Can you work these out from the model? Positions are in its coordinate system, mm. A direction names the side the tool comes from. Give positions to 0.01 mm unless a question says otherwise; leave off trailing zeros. Order: outer loops, then holes, each group sorted by start corner. A loop starts at its lowest first (then second) coordinate and runs counter-clockwise, first axis right, second up.
```python
from build123d import *

# Parameters (mm, degrees)
F2_R = 3.875


with BuildPart() as f3:
    # F3: sweep along a path in F0
    with BuildLine(Plane.XZ) as f3_path:
        Line((18, 62), (18, 16.4454190283))
        ThreePointArc((18, 16.4454190283), (17.4915763011, 14.2486617975), (16.0697030676, 12.4986579414))
        Line((16.0697030676, 12.4986579414), (3.0697030676, 2.3875468303))
        ThreePointArc((3.0697030676, 2.3875468303), (0, 1.3343079172), (-3.0697030676, 2.3875468303))
        Line((-3.0697030676, 2.3875468303), (-16.0697030676, 12.4986579414))
        ThreePointArc((-16.0697030676, 12.4986579414), (-17.4915763011, 14.2486617975), (-18, 16.4454190283))
        Line((-18, 16.4454190283), (-18, 62))
    # F2 (on offset) → F3 (sweep)
    with BuildSketch(Plane.XY.offset(62)):
        with Locations((18, 0)):
            Circle(F2_R)
    sweep(path=f3_path.line)


solid = f3.part
```
1) I'm going to push flat-ended pins straight in: pin 1 Ø4 at (x, y) = (-2.5, 0) entering from +Z; pin 2 Ø2 at (x, y) = (-13, -2.5) entering from -Z. Where does each tip first touch, or does it pass through?
2) If I drill on line 1 (X direction, y = 0, z = 25.5) (3 decimals); line 2 (X direction, y = 2, z = 17.5); line 3 (Z direction, x = 20.5, y = 1), over which ranges is the centre line in solid material (lowest first)?
3) Suppose I cut it at B-B (y = 0). Please give me the cut outline in (x, z) (3 decimals).
4) Suppose I cut it at A-A (z = 41). Please give me the cut outline in (x, y) (3 decimals).
5) Which directions (+Z, -Z, +X, -X, +Y, -Y) give clear straight access to the entire face, cutting with the end or side of a thin tool? Please do faces 1 (the face through (-14.13, -0.17, 39.54)), 2 (the face through (9.169, -3.842, 7.771)).
6) We'd pull the mould along X, two halves only. Please class faces 3 (the face through (-9.351, -3.842, 7.912)), 4 (the face through (-18, 0, 62)): +X half, -X half, draft (parallel to the pull), parting line (faces both ways), or undercut.
Results:
1. pin 1: stops at z = 8.41
1. pin 2: stops at z = 5.21
2. line 1: x = -21.875 to -14.125, 14.125 to 21.875
2. line 2: x = -21.32 to -14.68, 14.68 to 21.32
2. line 3: z = 11.95 to 62
3. outline: (-21.875, 16.445) arc R8.875 ccw to (-18.449, 9.44) - (-5.449, -0.671) arc R8.875 ccw to (5.449, -0.671) - (18.449, 9.44) arc R8.875 ccw to (21.875, 16.445) - (21.875, 62) - (14.125, 62) - (14.125, 16.445) arc R1.125 cw to (13.691, 15.557) - (0.691, 5.446) arc R1.125 cw to (-0.691, 5.446) - (-13.691, 15.557) arc R1.125 cw to (-14.125, 16.445) - (-14.125, 62) - (-21.875, 62) - close
4. outline: circle Ø7.75 at (-18, 0); circle Ø7.75 at (18, 0)
5. face 1: +Z
5. face 2: none
6. face 3: undercut
6. face 4: draft
